Can you work these out from the model? Positions are in its coordinate system, mm. Face numbers are marked on the shaded views. Coordinates: 2 decimals unless noted, no trailing zeros. Loops run counter-clockwise (first coordinate to the right, second up) from the corner with the lowest first, then second, coordinate; pieces in that order, holes last. Notation, with made-up numbers: (29, -25.75) -> (60, -25.75) arc R22 cw to (60, -18.75) -> close; hole circle Ø9 at (42, 58). An arc over 180 degrees is marked (long way). Put each result on its own line as item: value. Start each with the question number.
Item 1: If we section it at C-C on z = 13.5: Please give me the cut outline in (x, y), plus the area to 3 significant figures.
Item 2: If we section it at D-D on x = 1.5: Please give me the cut outline in (y, z).
Item 3: We'd pull the mould along X, two halves only. Please class the marked faces 1 and 2: pulls with the +X half, pulls with the -X half, needs draft (parallel to the pull), parting line crosses it, or undercut.
Item 4: If we section it at B-B on x = 0: Please give me the cut outline in (y, z).
Item 5: Will this pin go through, and if not, where does the flat tip stop? P1, Ø3, axis at x = 0, z = -13.5, coming from the +Y side.
Item 6: If we section it at A-A on y = 2: Please give me the cut outline in (x, z), plus the area to 3 significant figures.
Item 7: Please list where these lines run through material, in increasing order: L1, parallel to Z at x = 0, y = 2; L2, parallel to X at y = 2.35, z = -13.5; L3, parallel to Z at x = 1.25, y = 1.7. Write a range as from..to.
Autodesk Inventor part; units mm, degrees
ref_plane "YZ Plane" through (0, 0, 0) normal (1, 0, 0) x (0, 1, 0)
ref_plane "XZ Plane" through (0, 0, 0) normal (0, 1, 0) x (-1, 0, 0)
ref_plane "XY Plane" through (0, 0, 0) normal (0, 0, 1) x (1, 0, 0)
sketch "Sketch1" plane through (0, 0, 0) normal (0, 1, 0) x (-1, 0, 0)
  line L0 (-4, 20) -> (4, 20)
  line L1 (4, 20) -> (4, -20)
  line L2 (4, -20) -> (-4, -20)
  line L3 (-4, -20) -> (-4, 20)
  line L4 (-4, 20) -> (4, -20) construction
  line L5 (4, 20) -> (-4, -20) construction
  line L6 (0, -20) -> (0, -13.5) construction
  line L7 (0, 20) -> (0, 13.5) construction
  point P0 (0, 0)
  dimension "d0" = 40
  dimension "d1" = 6.5
  dimension "d2" = 8
extrude "Extrusion1" add sketch "Sketch1" along normal blind 3
hole "Hole1" at (0, 0, -13.5) at (0, 0, 13.5) direction (0, 1, 0) diameter 4 end through all
fillet "Fillet1" radius 1 4 edges at (4, 1.5, 20) (-4, 1.5, 20) (4, 1.5, -20) (-4, 1.5, -20)
equation "\"d0\" = gauge_length"
equation "\"d1\" = hole_2_border"
equation "\"d2\" = gauge_width"
equation "\"d3\" = gauge_thickness"
equation "\"d5\" = hole_diameter"
equation "\"gauge_length\" = 40"
equation "\"gauge_width\" = 8"
equation "\"gauge_thickness\" = 3"
equation "\"hole_diameter\" = 4"
equation "\"hole_2_border\" = 6.5"
properties part number "gauge" material "Stainless Steel"
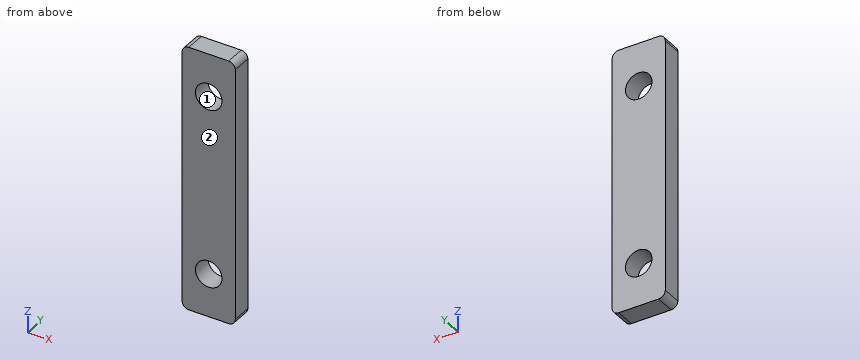
Solutions:
1. outline: (-4, 0) -> (-2, 0) -> (-2, 3) -> (-4, 3) -> close; (2, 0) -> (4, 0) -> (4, 3) -> (2, 3) -> close
1. area: 12.0 mm^2
2. outline: (0, -20) -> (3, -20) -> (3, -14.82) -> (0, -14.82) -> close; (0, -12.18) -> (3, -12.18) -> (3, 12.18) -> (0, 12.18) -> close; (0, 14.82) -> (3, 14.82) -> (3, 20) -> (0, 20) -> close
3. face 1: undercut
3. face 2: needs draft
4. outline: (0, -20) -> (3, -20) -> (3, -15.5) -> (0, -15.5) -> close; (0, -11.5) -> (3, -11.5) -> (3, 11.5) -> (0, 11.5) -> close; (0, 15.5) -> (3, 15.5) -> (3, 20) -> (0, 20) -> close
5. P1: through
6. outline: (-4, -19) arc R1 ccw to (-3, -20) -> (3, -20) arc R1 ccw to (4, -19) -> (4, 19) arc R1 ccw to (3, 20) -> (-3, 20) arc R1 ccw to (-4, 19) -> close; hole circle Ø4 at (0, -13.5); hole circle Ø4 at (0, 13.5)
6. area: 294 mm^2
7. L1: -20..-15.5, -11.5..11.5, 15.5..20
7. L2: -4..-2, 2..4
7. L3: -20..-15.06, -11.94..11.94, 15.06..20
